The model under review builds one solid part; all positions refer to its coordinate system, in mm. Face numbers are marked on the shaded views. A direction names the side the tool comes from. Give positions to 0.01 mm unless a question says otherwise; leave off trailing zeros. Write each loop counter-clockwise with the first axis right and the second up, starting at its lowest first coordinate (ties: lowest second). Pieces come first, ordered by that corner, then holes. Notation, with made-up numbers: (-37.75, 75) - (-2.75, 75) arc R28 cw to (-2.75, 97) - close; hole circle Ø8 at (70.25, 68). An arc over 180 degrees is marked (long way). Write item = value, one per line.
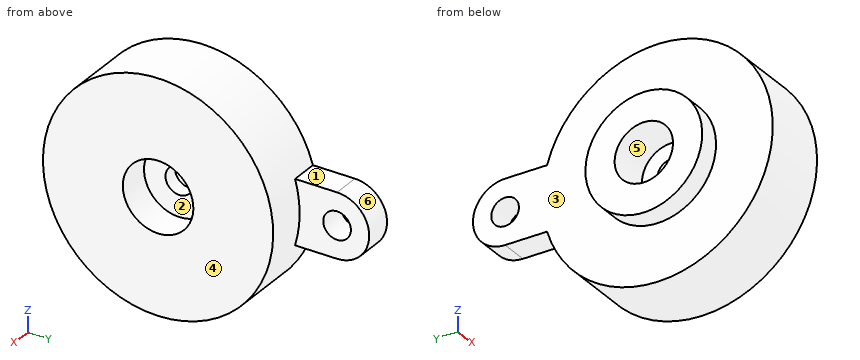
```python
from build123d import *

# Parameters (mm, degrees)
SKETCH1_R           = 12.075
BOSS_EXTRUDE1_DEPTH = 3.6
BOSS_EXTRUDE2_DEPTH = 2.9
SKETCH3_R           = 6.125
BOSS_EXTRUDE3_DEPTH = 2.25
SKETCH4_R           = 3.0625
CUT_EXTRUDE1_DEPTH  = 4.44
SKETCH5_R           = 1.45
CUT_EXTRUDE2_DEPTH  = 24.372983335
SKETCH6_R           = 3.7
CUT_EXTRUDE3_DEPTH  = 3.45
SKETCH7_R           = 1.45
CUT_EXTRUDE4_DEPTH  = 24.938175578


with BuildPart() as part:
    # Sketch1 → Boss-Extrude1 (new, symmetric)
    with BuildSketch(Plane(origin=(0, 0, 0), x_dir=(0, 0, -1), z_dir=(1, 0, 0))):
        Circle(SKETCH1_R)
    extrude(amount=BOSS_EXTRUDE1_DEPTH, both=True)

    # Sketch2 → Boss-Extrude2 (add)
    with BuildSketch(Plane.ZY.offset(3.6)):
        with BuildLine():
            Line((-3.375, 0), (-3.375, 16))
            ThreePointArc((-3.375, 16), (0, 19.375), (3.375, 16))
            Line((3.375, 16), (3.375, 0))
            ThreePointArc((3.375, 0), (0, -3.375), (-3.375, 0))
        make_face()
    extrude(amount=-BOSS_EXTRUDE2_DEPTH)

    # Sketch3 → Boss-Extrude3 (add)
    with BuildSketch(Plane.ZY.offset(3.6)):
        Circle(SKETCH3_R)
    extrude(amount=BOSS_EXTRUDE3_DEPTH)

    # Sketch4 → Cut-Extrude1 (cut)
    with BuildSketch(Plane.ZY.offset(5.85)):
        Circle(SKETCH4_R)
    extrude(amount=-CUT_EXTRUDE1_DEPTH, mode=Mode.SUBTRACT)

    # Sketch5 → Cut-Extrude2 (cut, through all)
    with BuildSketch(Plane.ZY.offset(1.41)):
        Circle(SKETCH5_R)
    extrude(amount=-CUT_EXTRUDE2_DEPTH, mode=Mode.SUBTRACT)

    # Sketch6 → Cut-Extrude3 (cut)
    with BuildSketch(Plane(origin=(3.6, 0, 0), x_dir=(0, 0, -1), z_dir=(1, 0, 0))):
        Circle(SKETCH6_R)
    extrude(amount=-CUT_EXTRUDE3_DEPTH, mode=Mode.SUBTRACT)

    # Sketch7 → Cut-Extrude4 (cut, through all)
    with BuildSketch(Plane.ZY.offset(3.6)):
        with Locations((0, 16)):
            Circle(SKETCH7_R)
    extrude(amount=-CUT_EXTRUDE4_DEPTH, mode=Mode.SUBTRACT)


solid = part.part
```
1. For line 1 (Y direction, x = 1, z = -0.25); line 2 (Y direction, x = -3.8, z = 0) (1 decimal); line 3 (X direction, y = 8.5, z = -3.5), list the stretches that pass through material, from the lowest coordinate up. Write a range as from..to.
Findings below:
line_1 = -12.07..-3.69, 3.69..12.07
line_2 = -6.1..-3.1, 3.1..6.1
line_3 = -3.6..3.6
2. Insertion check: P1, Ø3.5, axis at y = 0, z = 0.5, coming from the +X side; P2, Ø5, axis at x = 1.5, y = -8.5, coming from the -Z side; P3, Ø1.8, axis at y = -0.5, z = -0.5, coming from the -X side. Each pin has a flat end and moves straight along its axis. Give the tip position at first contact, or say it passes through.
Findings below:
P1 = 0.15
P2 = -10.48
P3 = -1.41
3. Draft analysis for pull direction Y (two halves, no side actions). For the marked faces 4, 5 and 6, state which applies: +Y half, -Y half, draft (parallel to the pull), parting line (faces both ways), or undercut.
Findings below:
face_4 = draft
face_5 = undercut
face_6 = +Y half
4. Take a section at D-D on x = 0.5. Give the boundary of the cut face in (y, z) (3 decimals).
Findings below:
outline = circle Ø24.15 at (0, 0); hole circle Ø7.4 at (0, 0)
5. Machinability: for the marked faces 1, 2 and 3, which of the approach directions +Z, -Z, +X, -X, +Y, -Y give a long, thin tool a straight path to every point of the face, cutting with its end or side? Answer none if there is none.
Findings below:
face_1 = +Z, +X, -X, +Y
face_2 = +X
face_3 = -X
6. Take a section at B-B on z = 0. Count the separate pieces of the cut face and the enclosed holes in it, and give its area (3 significant figures).
Findings below:
separate_pieces = 3
enclosed_holes = 0
area = 157 mm²
